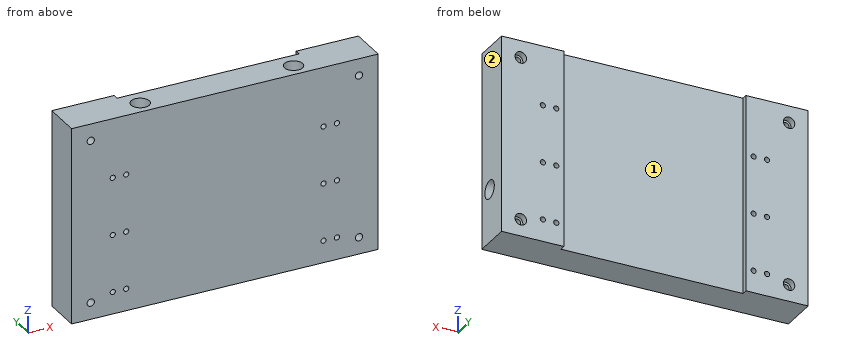
from build123d import *

# Parameters (mm, degrees)
SKETCH1_W                                      = 160.02
SKETCH1_H                                      = 102.616
BODY_DEPTH                                     = 19.9898
CBORE_FOR_6_SOCKET_HEAD_CAP_SCREW1_D           = 3.7973
CBORE_FOR_6_SOCKET_HEAD_CAP_SCREW1_CBORE_D     = 5.9944
CBORE_FOR_6_SOCKET_HEAD_CAP_SCREW1_CBORE_DEPTH = 3.683
TAP_DRILL_FOR_6_32_TAP1_D                      = 2.7051
SKETCH6_W                                      = 95
SKETCH6_H                                      = 102.616
GOUGE_DEPTH                                    = 2.9972
SKETCH7_R                                      = 4.572
PIPES1_DEPTH                                   = 80.01
SKETCH8_R                                      = 4.572
PIPES2_DEPTH                                   = 119.888
PIPE_TAP_DRILL_FOR_1_8_TAP2_D                  = 9.525
PIPE_TAP_DRILL_FOR_1_8_TAP2_DEPTH              = 20.066
PIPE_TAP_DRILL_FOR_1_8_TAP2_TIP                = 2.861598698
PIPE_TAP_DRILL_FOR_1_8_TAP3_D                  = 9.525
PIPE_TAP_DRILL_FOR_1_8_TAP3_DEPTH              = 20.066
PIPE_TAP_DRILL_FOR_1_8_TAP3_TIP                = 2.861598698


with BuildPart() as part:
    # Sketch1 → body (new body)
    with BuildSketch(Plane(origin=(0, 0, 0), x_dir=(1, 0, 0), z_dir=(0, 1, 0))):
        with Locations((80.01, 51.308)):
            Rectangle(SKETCH1_W, SKETCH1_H)
    extrude(amount=BODY_DEPTH)

    # CBORE for #6 Socket Head Cap Screw1 (through all)
    with Locations(Plane(origin=(0, 19.9898, 0), x_dir=(1, 0, 0), z_dir=(0, 1, 0))):
        with Locations((10.0076, 93.8276), (150.0124, 8.8138), (10.0076, 8.8138), (150.0124, 93.8276)):
            CounterBoreHole(CBORE_FOR_6_SOCKET_HEAD_CAP_SCREW1_D / 2, CBORE_FOR_6_SOCKET_HEAD_CAP_SCREW1_CBORE_D / 2, CBORE_FOR_6_SOCKET_HEAD_CAP_SCREW1_CBORE_DEPTH)

    # Tap Drill for #6-32 Tap1 (through all)
    with Locations(Plane(origin=(0, 19.9898, 0), x_dir=(1, 0, 0), z_dir=(0, 1, 0))):
        with Locations((28.5, 91.0844), (28.5, 31.0844), (28.5, 61.0844), (131.5, 91.0844), (131.5, 31.0844), (131.5, 61.0844), (21.5, 91.0844), (21.5, 61.0844), (21.5, 31.0844), (138.5, 31.0844), (138.5, 61.0844), (138.5, 91.0844)):
            Hole(TAP_DRILL_FOR_6_32_TAP1_D / 2)

    # Sketch6 → gouge (cut)
    with BuildSketch(Plane(origin=(0, 19.9898, 0), x_dir=(1, 0, 0), z_dir=(0, 1, 0))):
        with Locations((80.012, 51.308)):
            Rectangle(SKETCH6_W, SKETCH6_H)
    extrude(amount=-GOUGE_DEPTH, mode=Mode.SUBTRACT)

    # Sketch7 → pipes1 (cut)
    with BuildSketch(Plane.XY):
        with Locations((39.878, 7.874)):
            Circle(SKETCH7_R)
        with Locations((119.888, 7.874)):
            Circle(SKETCH7_R)
    extrude(amount=-PIPES1_DEPTH, mode=Mode.SUBTRACT)

    # Sketch8 → pipes2 (cut)
    with BuildSketch(Plane(origin=(160.02, 0, 0), x_dir=(0, 0, -1), z_dir=(1, 0, 0))):
        with Locations((74.93, 7.874)):
            Circle(SKETCH8_R)
    extrude(amount=-PIPES2_DEPTH, mode=Mode.SUBTRACT)

    # Pipe Tap Drill for 1/8 Tap2
    with Locations(Plane.XY):
        with Locations((39.878, 7.874), (119.888, 7.874)):
            Hole(PIPE_TAP_DRILL_FOR_1_8_TAP2_D / 2, depth=PIPE_TAP_DRILL_FOR_1_8_TAP2_DEPTH)
            with Locations((0, 0, -(PIPE_TAP_DRILL_FOR_1_8_TAP2_DEPTH + PIPE_TAP_DRILL_FOR_1_8_TAP2_TIP / 2))):  # 118° drill point
                Cone(0, PIPE_TAP_DRILL_FOR_1_8_TAP2_D / 2, PIPE_TAP_DRILL_FOR_1_8_TAP2_TIP, mode=Mode.SUBTRACT)

    # Pipe Tap Drill for 1/8 Tap3
    with Locations(Plane(origin=(160.02, 0, 0), x_dir=(0, 0, -1), z_dir=(1, 0, 0))):
        with Locations((74.93, 7.874)):
            Hole(PIPE_TAP_DRILL_FOR_1_8_TAP3_D / 2, depth=PIPE_TAP_DRILL_FOR_1_8_TAP3_DEPTH)
            with Locations((0, 0, -(PIPE_TAP_DRILL_FOR_1_8_TAP3_DEPTH + PIPE_TAP_DRILL_FOR_1_8_TAP3_TIP / 2))):  # 118° drill point
                Cone(0, PIPE_TAP_DRILL_FOR_1_8_TAP3_D / 2, PIPE_TAP_DRILL_FOR_1_8_TAP3_TIP, mode=Mode.SUBTRACT)


solid = part.part
Input: part model. Units: mm. Frame: model coordinates. Face numbers are marked on the shaded views. A direction names the side the tool comes from. Give positions to 0.01 mm unless a question says otherwise; leave off trailing zeros. Loops run counter-clockwise (first coordinate to the right, second up) from the corner with the lowest first, then second, coordinate; pieces in that order, holes last. Notation, with made-up numbers: M 79,17 L 89,17 A26 ccw 89,35 Z; hole C -24.5,47 d2. An arc over 180 degrees is marked long. Use one line per item in the form item = value.
1. Section query C-C, the plane x = 70. Return the cut outline in (y, z).
Numbers:
outline = M 0,-102.62 L 16.99,-102.62 L 16.99,0 L 0,0 Z; hole C 7.87,-74.93 d9.14
2. Line query: L1, parallel to Z at x = 131.5, y = 15.25; L2, parallel to X at y = 7.5, z = -35; L3, parallel to Y at x = 129.5, z = -74.93. Output: solid intervals per line, ascending.
Numbers:
L1 = -102.62 to -92.44, -89.73 to -62.44, -59.73 to -32.44, -29.73 to 0
L2 = 0 to 35.32, 44.43 to 115.33, 124.44 to 160.02
L3 = 0 to 3.3, 12.45 to 19.99
3. Section query A-A, the plane z = -82. Return the cut outline in (x, y), and give its area (3 significant figures).
Numbers:
outline = M 0,0 L 160.02,0 L 160.02,19.99 L 127.51,19.99 L 127.51,16.99 L 32.51,16.99 L 32.51,19.99 L 0,19.99 Z
area = 2,910 mm²
4. Reachability of the marked faces 1 and 2 from +Z, -Z, +X, -X, +Y, -Y: full face, straight path, thin tool, end or side. Return the list, or none.
Numbers:
face_1 = +Z, -Z, +Y
face_2 = +Z, -Z, +X, +Y, -Y
5. First-contact query: pin 1 (7.5 mm diameter, centred on x = 39, y = 6.5, fed in from +Z); pin 2 (1.8 mm diameter, centred on x = 149, z = -93, fed in from +Y); pin 3 (7.5 mm diameter, centred on x = 119.888, y = 7.874, fed in from +Z); pin 4 (12 mm diameter, centred on x = 90, z = -31, fed in from +Y). Flat tips, straight axial feed; report the tip coordinate or a pass-through.
Numbers:
pin_1 = 0
pin_2 = 16.31
pin_3 = -80.01
pin_4 = 16.99
6. Section query B-B, the plane z = -38. Return the cut outline in (x, y), and give its area (3 significant figures).
Numbers:
outline = M 0,0 L 160.02,0 L 160.02,19.99 L 127.51,19.99 L 127.51,16.99 L 32.51,16.99 L 32.51,19.99 L 0,19.99 Z; hole C 39.88,7.87 d9.14; hole C 119.89,7.87 d9.14
area = 2,780 mm²
